Model file for the job. Use its own axes, mm. Coordinates: 2 decimals unless noted, no trailing zeros. Order: outer loops, then holes, each group sorted by start corner. A loop starts at its lowest first (then second) coordinate and runs counter-clockwise, first axis right, second up.
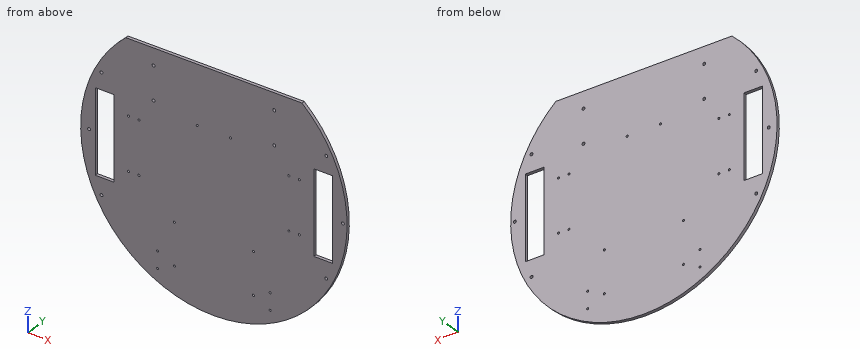
Autodesk Inventor part; units mm, degrees
ref_plane "YZ Plane" through (0, 0, 0) normal (1, 0, 0) x (0, 1, 0)
ref_plane "XZ Plane" through (0, 0, 0) normal (0, 1, 0) x (-1, 0, 0)
ref_plane "XY Plane" through (0, 0, 0) normal (0, 0, 1) x (1, 0, 0)
sketch "Sketch1" plane through (0, 0, 0) normal (0, 1, 0) x (-1, 0, 0)
  circle A0 centre (0, 0) radius 203.2
  dimension "d0" = 406.4
extrude "Extrusion1" add sketch "Sketch1" along normal blind 4.7625
sketch "Sketch2" plane through (0, 4.7625, 0) normal (0, 1, 0) x (1, 0, 0)
  point P0 (0, 0)
  point P1 (114.3, 40.005)
  point P2 (114.3, -39.995)
  point P3 (-114.3, 40.005)
  point P4 (-114.3, -39.995)
  dimension "d3" = 0
  dimension "d4" = 80
  dimension "d5" = 40.005
  dimension "d6" = 0
  dimension "d7" = 0
  dimension "d8" = 0
  dimension "d9" = 114.3
  dimension "d10" = 114.3
hole "Hole1" at (114.3, 4.7625, -40.005) at (114.3, 4.7625, 39.995) at (-114.3, 4.7625, -40.005) at (-114.3, 4.7625, 39.995) direction (0, -1, 0) diameter 3.175 end through all
sketch "Sketch3" plane through (0, 4.7625, 0) normal (0, 1, 0) x (1, 0, 0)
  line L0 (180.975, 63.5) -> (152.4, 63.5)
  line L1 (152.4, 63.5) -> (152.4, -63.5)
  line L2 (152.4, -63.5) -> (180.975, -63.5)
  line L3 (180.975, -63.5) -> (180.975, 63.5)
  line L4 (-152.4, 63.5) -> (-180.975, 63.5)
  line L5 (-180.975, 63.5) -> (-180.975, -63.5)
  line L6 (-180.975, -63.5) -> (-152.4, -63.5)
  line L7 (-152.4, -63.5) -> (-152.4, 63.5)
  point P0 (0, 0)
  dimension "d18" = 0
  dimension "d19" = 0
  dimension "d20" = 152.4
  dimension "d21" = 152.4
  dimension "d22" = 127
  dimension "d23" = 63.5
  dimension "d24" = 28.575
  dimension "d25" = 28.575
extrude "Extrusion2" cut sketch "Sketch3" against normal blind 25.4
sketch "Sketch4" plane through (0, 4.7625, 0) normal (0, 1, 0) x (1, 0, 0)
  line L0 (152.4, -63.5) -> (152.4, 63.5)
  line L1 (152.4, 63.5) -> (180.975, 63.5)
  line L2 (180.975, 63.5) -> (180.975, -63.5)
  line L3 (180.975, -63.5) -> (152.4, -63.5)
  line L4 (-180.975, -63.5) -> (-180.975, 63.5)
  line L5 (-180.975, 63.5) -> (-152.4, 63.5)
  line L6 (-152.4, 63.5) -> (-152.4, -63.5)
  line L7 (-152.4, -63.5) -> (-180.975, -63.5)
  circle A0 centre (-114.3, 40.005) radius 1.5875
  circle A1 centre (114.3, 40.005) radius 1.5875
  circle A2 centre (114.3, -39.995) radius 1.5875
  circle A3 centre (-114.3, -39.995) radius 1.5875
  circle A4 centre (0, 0) radius 203.2
  circle A5 centre (114.3, -39.995) radius 1.5875
  point P0 (-130.302, 40.005)
  point P1 (-130.302, -39.995)
  point P2 (130.302, 40.005)
  point P3 (130.302, -39.995)
  dimension "d28" = 0
  dimension "d29" = 0
  dimension "d30" = 0
  dimension "d32" = 0
  dimension "d33" = 0
  dimension "d34" = 0
  dimension "d43" = 16.002
  dimension "d44" = 16.002
hole "Hole2" at (-130.302, 4.7625, -40.005) at (-130.302, 4.7625, 39.995) at (130.302, 4.7625, -40.005) at (130.302, 4.7625, 39.995) direction (0, -1, 0) diameter 3.175 end through all
sketch "Sketch5" plane through (0, 4.7625, 0) normal (0, 1, 0) x (1, 0, 0)
  point P0 (0, 0)
  point P1 (60.325, 152.4)
  point P2 (60.325, 88.9)
  point P3 (-60.325, 88.9)
  point P4 (-60.325, 152.4)
  dimension "d45" = 0
  dimension "d46" = 0
  dimension "d47" = 0
  dimension "d48" = 0
  dimension "d49" = 60.325
  dimension "d50" = 60.325
  dimension "d51" = 63.5
  dimension "d52" = 88.9
hole "Hole3" at (60.325, 4.7625, -152.4) at (60.325, 4.7625, -88.9) at (-60.325, 4.7625, -88.9) at (-60.325, 4.7625, -152.4) direction (0, -1, 0) diameter 3.175 end through all
sketch "Sketch6" plane through (0, 4.7625, 0) normal (0, 1, 0) x (1, 0, 0)
  circle A0 centre (60.325, 152.4) radius 1.5875
  circle A1 centre (-60.325, 152.4) radius 1.5875
  point P0 (0, 0)
  point P1 (-85.725, 139.7)
  point P2 (85.725, 139.7)
  point P3 (-85.725, 165.1)
  point P4 (85.725, 165.1)
  dimension "d64" = 0
  dimension "d65" = 25.4
  dimension "d66" = 0
  dimension "d67" = 25.4
  dimension "d68" = 12.7
  dimension "d69" = 25.4
  dimension "d70" = 12.7
  dimension "d71" = 25.4
hole "Hole4" at (-85.725, 4.7625, -139.7) at (85.725, 4.7625, -139.7) at (-85.725, 4.7625, -165.1) at (85.725, 4.7625, -165.1) direction (0, -1, 0) diameter 3.175 end through all
sketch "Sketch8" plane through (0, 4.7625, 0) normal (0, 1, 0) x (1, 0, 0)
  line L0 (-76.2, 0) -> (-76.2, -101.6)
  line L1 (-76.2, -101.6) -> (76.2, -101.6)
  point P0 (0, 0)
  point P1 (-25.4, -63.5)
  point P2 (25.4, -63.5)
  point P3 (-203.2, 0)
  dimension "d86" = 0
  dimension "d89" = 50.8
  dimension "d99" = 63.5
  dimension "d100" = 25.4
hole "Hole5" at (-25.4, 4.7625, 63.5) at (25.4, 4.7625, 63.5) direction (0, -1, 0) diameter 3.175 depth 25.4 tip angle 118.188
sketch "Sketch9" plane through (0, 4.7625, 0) normal (0, 1, 0) x (1, 0, 0)
  line L0 (-76.2, -158.75) -> (76.2, -158.75)
  line L1 (76.2, -158.75) -> (76.2, -299.4145)
  line L2 (76.2, -299.4145) -> (-76.2, -299.4145)
  line L3 (-76.2, -299.4145) -> (-76.2, -158.75)
  point P0 (0, 0)
  dimension "d101" = 158.75
  dimension "d104" = 76.2
  dimension "d105" = 76.2
extrude "Extrusion4" cut sketch "Sketch9" against normal blind 25.4
sketch "Sketch10" plane through (0, 4.7625, 0) normal (0, 1, 0) x (1, 0, 0)
  circle A0 centre (25.4, -63.5) radius 1.5875
  point P0 (0, 0)
  point P1 (-92.075, -76.2)
  point P2 (-92.075, -127)
  point P3 (92.075, -76.2)
  point P4 (92.075, -127)
  dimension "d106" = 0
  dimension "d107" = 0
  dimension "d108" = 0
  dimension "d109" = 50.8
  dimension "d110" = 0
  dimension "d111" = 92.075
  dimension "d112" = 92.075
  dimension "d113" = 12.7
hole "Hole6" at (-92.075, 4.7625, 76.2) at (-92.075, 4.7625, 127) at (92.075, 4.7625, 76.2) at (92.075, 4.7625, 127) direction (0, -1, 0) diameter 4.4958 end through all
sketch "Sketch11" plane through (0, 4.7625, 0) normal (0, 1, 0) x (1, 0, 0)
  line L0 (-208.3866, -152.4) -> (200.3636, -152.4)
  line L1 (200.3636, -152.4) -> (200.3636, -247.6891)
  line L2 (200.3636, -247.6891) -> (-208.3866, -247.6891)
  line L3 (-208.3866, -247.6891) -> (-208.3866, -152.4)
  circle A0 centre (-92.075, -127) radius 2.2479
  point P0 (0, 0)
  dimension "d121" = 25.4
extrude "Extrusion5" cut sketch "Sketch11" against normal blind 25.4 contours L0 L1 L2 L3
sketch "Sketch12" plane through (0, 4.7625, 0) normal (0, 1, 0) x (1, 0, 0)
  point P0 (0, 0)
  point P1 (196.85, 0)
  point P2 (171.45, 88.9)
  point P3 (171.45, -88.9)
  point P4 (-171.45, -88.9)
  point P5 (-190.5, 0)
  point P6 (-171.45, 88.9)
  dimension "d124" = 0
  dimension "d125" = 88.9
  dimension "d126" = 88.9
  dimension "d127" = 171.45
  dimension "d128" = 171.45
  dimension "d129" = 171.45
  dimension "d130" = 171.45
  dimension "d131" = 88.9
  dimension "d132" = 88.9
  dimension "d133" = 0
  dimension "d134" = 196.85
  dimension "d142" = 190.5
hole "Hole7" at (196.85, 4.7625, 0) at (171.45, 4.7625, -88.9) at (171.45, 4.7625, 88.9) at (-171.45, 4.7625, 88.9) at (-190.5, 4.7625, 0) at (-171.45, 4.7625, -88.9) direction (0, -1, 0) diameter 4.4958 end through all
properties part number "BottomPlate"
Q1. Cut at A-A, the plane y = 2.45. Count the separate pieces of the cut face and the enclosed holes in it, plus the area to 3 significant figures.
Established:
separate pieces: 1
enclosed holes: 30
area: 113,000 mm2
Q2. Probe line 1 (X direction, y = 2.6, z = 0) (3 decimals); line 2 (X direction, y = 3.7, z = -6) (3 decimals); line 3 (X direction, y = 1.85, z = 55) (3 decimals). List the from-to ranges inside material, lowest first.
Established:
line 1: x = -203.2 to -192.748, -188.252 to -180.975, -152.4 to 152.4, 180.975 to 194.602, 199.098 to 203.2
line 2: x = -203.111 to -180.975, -152.4 to 152.4, 180.975 to 203.111
line 3: x = -195.615 to -180.975, -152.4 to 152.4, 180.975 to 195.615
Q3. Drop flat-ended pins along their axis: P1, Ø1.4, axis at y = 1.5, z = 24.5, coming from the +X side; P2, Ø2, axis at x = 152, y = 3.5, coming from the -Z side. Give the stop position or say it passes through.
Established:
P1: stops at x = 201.8
P2: stops at z = -135.98
Q4. Cut at B-B, the plane x = -103. List the corners of the cut face in (y, z), plus the area to 3 significant figures.
Established:
outline: (0, -175.16) - (4.76, -175.16) - (4.76, 152.4) - (0, 152.4) - close
area: 1,560 mm2
Q5. Cut at C-C, the plane x = 72.5. List the corners of the cut face in (y, z), plus the area to 3 significant figures.
Established:
outline: (0, -189.83) - (4.76, -189.83) - (4.76, 152.4) - (0, 152.4) - close
area: 1,630 mm2
